```python
from build123d import *

# Parameters (mm, degrees)
F1_DEPTH = 1
F3_DEPTH = 1
F4_R     = 2


with BuildPart() as f1:
    # F0 (on Front) → F1 (new body)
    with BuildSketch(Plane.XZ):
        with BuildLine():
            Line((-6, -10), (6, -10))
            Line((6, -10), (6, 4))
            ThreePointArc((6, 4), (4.242641, 8.242641), (0, 10))
            ThreePointArc((0, 10), (-4.242641, 8.242641), (-6, 4))
            Line((-6, 4), (-6, -10))
        make_face()
        with BuildLine():
            Line((2, 4), (2, -4))
            ThreePointArc((2, -4), (1.414214, -5.414214), (0, -6))
            ThreePointArc((0, -6), (-1.414214, -5.414214), (-2, -4))
            Line((-2, -4), (-2, 4))
            ThreePointArc((-2, 4), (-1.414214, 5.414214), (0, 6))
            ThreePointArc((0, 6), (1.414214, 5.414214), (2, 4))
        make_face(mode=Mode.SUBTRACT)
    extrude(amount=-F1_DEPTH)

    # F2 (on face) → F3 (join)
    with BuildSketch(Plane(origin=(0, 0, -10), x_dir=(1, 0, 0), z_dir=(0, 0, -1))):
        with BuildLine():
            Line((6, -1), (-6, -1))
            Line((-6, -1), (-6, -34))
            ThreePointArc((-6, -34), (-4.242641, -38.242641), (0, -40))
            ThreePointArc((0, -40), (4.242641, -38.242641), (6, -34))
            Line((6, -34), (6, -1))
        make_face()
        with BuildLine():
            Line((2, -7), (2, -33))
            ThreePointArc((2, -33), (1.414214, -34.414214), (0, -35))
            ThreePointArc((0, -35), (-1.414214, -34.414214), (-2, -33))
            Line((-2, -33), (-2, -7))
            ThreePointArc((-2, -7), (-1.414214, -5.585786), (0, -5))
            ThreePointArc((0, -5), (1.414214, -5.585786), (2, -7))
        make_face(mode=Mode.SUBTRACT)
    extrude(amount=-F3_DEPTH)

    # F4
    f4_edges = [f1.edges().sort_by_distance(p)[0] for p in [
        (0, 0, -10),
    ]]
    fillet(f4_edges, radius=F4_R)


solid = f1.part
```
Part model, mm, in its own coordinate system. A direction names the side the tool comes from. Round coordinates to 2 decimals unless told otherwise and drop trailing zeros. Order: outer loops, then holes, each group sorted by start corner. A loop starts at its lowest first (then second) coordinate and runs counter-clockwise, first axis right, second up. Notation, with made-up numbers: M 16,81.25 L 32,81.25 A19 ccw 32,99.25 Z; hole C -1,39 d8. An arc over 180 degrees is marked long. Put each result on its own line as item: value. Start each with the question number.
1. Two-plate mould, pull along Y, no slides. Class faces 4 (the face through (2, 19.8, -9.5)), 5 (the face through (-3, 21, -10)), 6 (the face through (0.08, 0.6, -9.43)), 7 (the face through (-2, 20.2, -9.5)): +Y half, -Y half, draft (parallel to the pull), parting line (faces both ways), or undercut.
2. Slice it at A-A on y = 12. List the corners of the cut face in (x, z), then the cut area to 3 significant figures.
3. Drop flat-ended pins along their axis: pin 1 (5 mm diameter, centred on x = -3, y = 34.5, fed in from +Z); pin 2 (4 mm diameter, centred on x = -0.5, z = 1.5, fed in from +Y). Give the stop position or say it passes through.
4. Slice it at C-C on x = -0.5. List the corners of the cut face in (y, z).
5. Slice it at B-B on z = 1.75. List the corners of the cut face in (x, y).
6. Drill centre lines: probe 1 along Z at (x, y) = (2.25, 38.5); probe 2 along Y at (x, z) = (-3.75, -1.5). Where is each one in solid material? Low to high. Write a range as [from, to].
7. Tool access for faces 1 (the face through (2, 0.5, 0.1)), 2 (the face through (6, 12, -9.3)), 3 (the face through (-3, 1, 1)): list every direction of +Z, -Z, +X, -X, +Y, -Y with a clear straight run to the whole face (end or side of a thin tool).
8. Slice it at D-D on x = 3.5. List the corners of the cut face in (y, z), then the cut area to 3 significant figures.
Findings:
1. face 4: undercut
1. face 5: draft
1. face 6: -Y half
1. face 7: undercut
2. outline: M -6,-10 L -2,-10 L -2,-9 L -6,-9 Z; M 2,-10 L 6,-10 L 6,-9 L 2,-9 Z
2. area: 8.00 mm2
3. pin 1: z = -9
3. pin 2: y = 1
4. outline: M 0,-8 A2 ccw 2,-10 L 5.06,-10 L 5.06,-9 L 1,-9 L 1,-5.94 L 0,-5.94 Z; M 0,5.94 L 1,5.94 L 1,9.98 L 0,9.98 Z; M 34.94,-10 L 39.98,-10 L 39.98,-9 L 34.94,-9 Z
5. outline: M -6,0 L -2,0 L -2,1 L -6,1 Z; M 2,0 L 6,0 L 6,1 L 2,1 Z
6. probe 1: [-10, -9]
6. probe 2: [0, 1]
7. face 1: +Y, -Y
7. face 2: +Z, -Z, +X, +Y, -Y
7. face 3: +Z, +X, -X, +Y
8. outline: M 0,-8 A2 ccw 2,-10 L 38.87,-10 L 38.87,-9 L 1,-9 L 1,8.87 L 0,8.87 Z
8. area: 55.9 mm2
